from build123d import *

# Parameters (mm, degrees)
CUT_EXTRUDE1_START = -20.6375
SKETCH3_R          = 49.1871
CUT_EXTRUDE1_DEPTH = 20.6375
FILLET3_R          = 3.175
CHAMFER1_SIZE      = 2.54
CUT_EXTRUDE2_DEPTH = 91.4621
CIRPATTERN1_COUNT  = 6


with BuildPart() as part:
    # Sketch2 → Revolve1 (revolve)
    with BuildSketch(Plane.XY):
        Polygon((-25.6794, 49.1871), (-6.6294, 49.1871), (-1.8669, 49.1871), (-1.8669, 46.105572), (1.8669, 46.105572), (1.8669, 49.1871), (4.7625, 49.1871), (4.7625, 34.0106), (-25.6794, 34.0106), align=None)
    revolve(axis=Axis((0, 0, 0), (1, 0, 0)))

    # Sketch3 → Cut-Extrude1 (cut)
    with BuildSketch(Plane.ZY.offset(25.6794).offset(CUT_EXTRUDE1_START)):
        Circle(SKETCH3_R)
        Polygon((0, 47.660264722), (41.275, 23.830132361), (41.275, -23.830132361), (0, -47.660264722), (-41.275, -23.830132361), (-41.275, 23.830132361), align=None, mode=Mode.SUBTRACT)
    extrude(amount=CUT_EXTRUDE1_DEPTH, mode=Mode.SUBTRACT)

    # Fillet3
    fillet3_edges = [part.edges().sort_by_distance(p)[0] for p in [
        (-15.36065, -23.830132361, 41.275),
        (-15.36065, 23.830132361, 41.275),
        (-15.36065, 47.660264722, 0),
        (-15.36065, 23.830132361, -41.275),
        (-15.36065, -23.830132361, -41.275),
        (-15.36065, -47.660264722, 0),
    ]]
    fillet(fillet3_edges, radius=FILLET3_R)

    # Chamfer1
    chamfer1_edges = [part.edges().sort_by_distance(p)[0] for p in [
        (4.7625, -34.0106, 0),
    ]]
    chamfer(chamfer1_edges, length=CHAMFER1_SIZE)

    # Sketch4 → Cut-Extrude2 (cut, through all)
    with BuildSketch(Plane(origin=(0, 0, -41.275), x_dir=(-1, 0, 0), z_dir=(0, 0, -1))):
        with BuildLine():
            Line((25.6794, -1.984502), (25.6794, 1.984502))
            Line((25.6794, 1.984502), (22.5044, 1.984502))
            ThreePointArc((22.5044, 1.984502), (20.519898, 0), (22.5044, -1.984502))
            Line((22.5044, -1.984502), (25.6794, -1.984502))
        make_face()
    cut_extrude2 = extrude(amount=-CUT_EXTRUDE2_DEPTH, mode=Mode.SUBTRACT)

    # CirPattern1: Cut-Extrude2 ×6 about axis
    cirpattern1_axis = Axis((0, 0, 0), (1, 0, 0))
    for i in range(1, CIRPATTERN1_COUNT):
        add(cut_extrude2.rotate(cirpattern1_axis, i * 360 / CIRPATTERN1_COUNT), mode=Mode.SUBTRACT)


solid = part.part
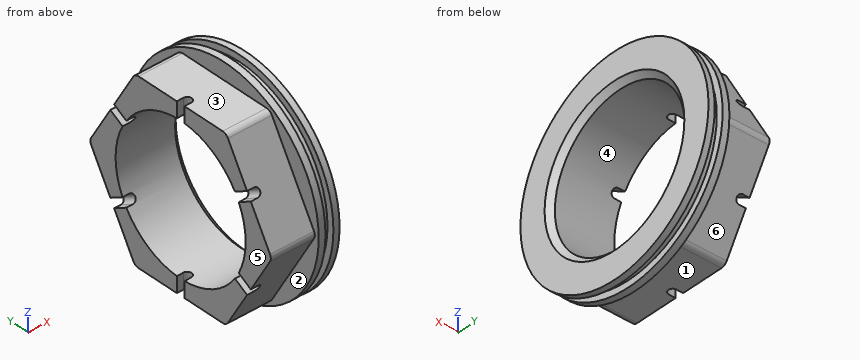
Verification items for the finished model (mm, model axes). Face numbers are marked on the shaded views. A direction names the side the tool comes from. Give positions to 0.01 mm unless a question says otherwise; leave off trailing zeros. Write each loop counter-clockwise with the first axis right and the second up, starting at its lowest first coordinate (ties: lowest second). Pieces come first, ordered by that corner, then holes.
(1) Material ranges on line 1 (Z direction, x = -7, y = 0) (3 decimals); line 2 (X direction, y = 31, z = -36); line 3 (Z direction, x = -5, y = 0), recorded low to high.
(2) Cross-section at D-D (y = 40). Enter the section's corners in (x, z).
(3) Mould release check, pull along Y, two halves, no side actions. Record for the marked faces 4, 5 and 6: +Y half, -Y half, draft (parallel to the pull), parting line (faces both ways), or undercut.
(4) Cross-section at A-A (y = 0). Enter the section's corners in (x, z) (1 decimal), plus the area to 3 significant figures.
(5) Access from +Z, -Z, +X, -X, +Y, -Y to the whole of each face (thin tool, end or side, straight path). Record for the marked faces 1, 2 and 3.
(6) Gauge pin test, flat ends, axial feed: pin 1 (2 mm diameter, centred on x = -20, z = 18.5, fed in from +Y); pin 2 (2 mm diameter, centred on x = -2.5, y = 24.5, fed in from +Z); pin 3 (12 mm diameter, centred on x = -7.5, y = 3.5, fed in from -Z); pin 4 (12 mm diameter, centred on y = -12, z = 25, fed in from +X). Record the tip position at first contact, or that the pin passes through.
(7) Cross-section at B-B (z = 0). Enter the section's corners in (x, y).
Worked out:
1. line 1: z = -41.275 to -34.011, 34.011 to 41.275
1. line 2: x = -5.04 to -1.87, 1.87 to 4.76
1. line 3: z = -49.19 to -34.01, 34.01 to 49.19
2. outline: (-25.68, -13.27) - (-5.04, -13.27) - (-5.04, -28.62) - (-1.87, -28.62) - (-1.87, -22.93) - (1.87, -22.93) - (1.87, -28.62) - (4.76, -28.62) - (4.76, 28.62) - (1.87, 28.62) - (1.87, 22.93) - (-1.87, 22.93) - (-1.87, 28.62) - (-5.04, 28.62) - (-5.04, 13.27) - (-25.68, 13.27) - close
3. face 4: undercut
3. face 5: draft
3. face 6: +Y half
4. outline: (-20.5, -41.3) - (-5, -41.3) - (-5, -49.2) - (-1.9, -49.2) - (-1.9, -46.1) - (1.9, -46.1) - (1.9, -49.2) - (4.8, -49.2) - (4.8, -36.6) - (2.2, -34) - (-20.5, -34) - close; (-20.5, 34) - (2.2, 34) - (4.8, 36.6) - (4.8, 49.2) - (1.9, 49.2) - (1.9, 46.1) - (-1.9, 46.1) - (-1.9, 49.2) - (-5, 49.2) - (-5, 41.3) - (-20.5, 41.3) - close
4. area: 493 mm2
5. face 1: -Z, -X, +Y, -Y
5. face 2: -X
5. face 3: +Z, -X, +Y, -Y
6. pin 1: stops at y = 37.56
6. pin 2: stops at z = 43.21
6. pin 3: stops at z = -49.19
6. pin 4: passes through
7. outline: (-25.68, -47.17) - (-5.04, -47.17) - (-5.04, -49.19) - (-1.87, -49.19) - (-1.87, -46.11) - (1.87, -46.11) - (1.87, -49.19) - (4.76, -49.19) - (4.76, -36.55) - (2.22, -34.01) - (-25.68, -34.01) - close; (-25.68, 34.01) - (2.22, 34.01) - (4.76, 36.55) - (4.76, 49.19) - (1.87, 49.19) - (1.87, 46.11) - (-1.87, 46.11) - (-1.87, 49.19) - (-5.04, 49.19) - (-5.04, 47.17) - (-25.68, 47.17) - close
